```python
from build123d import *

# Parameters (mm, degrees)
BOSS_EXTRU_1_DEPTH      = 5
ENL_V_MAT_EXTRU_1_REACH = 7


with BuildPart() as part:
    # Esquisse1 → Boss.-Extru.1 (new body)
    with BuildSketch(Plane.XY):
        Polygon((0, 0), (0, 15), (-5, 15), (-5, 55), (0, 55), (0, 80), (490, 80), (490, 55), (495, 55), (495, 15), (490, 15), (490, 0), align=None)
    extrude(amount=BOSS_EXTRU_1_DEPTH)

    # Esquisse2 → Enlèv. mat.-Extru.1 (cut, up to next)
    with BuildSketch(Plane.XY.offset(5), mode=Mode.PRIVATE) as enl_v_mat_extru_1_sk1:
        with BuildLine():
            Line((35, 25), (455, 25))
            ThreePointArc((455, 25), (462.071067812, 27.928932188), (465, 35))
            Line((465, 35), (465, 45))
            ThreePointArc((465, 45), (462.071067812, 52.071067812), (455, 55))
            Line((455, 55), (35, 55))
            ThreePointArc((35, 55), (27.928932188, 52.071067812), (25, 45))
            Line((25, 45), (25, 35))
            ThreePointArc((25, 35), (27.928932188, 27.928932188), (35, 25))
        make_face()
    enl_v_mat_extru_1_tool1 = extrude(enl_v_mat_extru_1_sk1.sketch, amount=-ENL_V_MAT_EXTRU_1_REACH, mode=Mode.PRIVATE) & part.part
    add(enl_v_mat_extru_1_tool1.solids().sort_by_distance((245, 40, 5))[0], mode=Mode.SUBTRACT)


solid = part.part
```
Verification items for the finished model (mm, model axes). A direction names the side the tool comes from. Round coordinates to 2 decimals unless told otherwise and drop trailing zeros. Loops run counter-clockwise (first coordinate to the right, second up) from the corner with the lowest first, then second, coordinate; pieces in that order, holes last. Notation, with made-up numbers: (84.25, 69) -> (136.25, 69) arc R34 ccw to (136.25, 103) -> close; hole circle Ø9 at (-18, 74). An arc over 180 degrees is marked (long way). Answer as a JSON object with one key per item and string values.
Q1. Draft check along Y on faces 3 (the cylindrical face through (462.15, 51.99, 2.54)), 4 (the flat face through (248, 58, 0)). Enter one of: pulls with the +Y half, pulls with the -Y half, needs draft (parallel to the pull), parting line crosses it, or undercut.
Data:
{"face 3": "undercut", "face 4": "needs draft"}
Q2. Scan lines: line 1 (X direction, y = 41, z = 2.5); line 2 (Y direction, x = 366.5, z = 4.1); line 3 (X direction, y = 65.5, z = 3.8). Record each from-to range of solid material in increasing order. Write a range as from..to.
Data:
{"line 1": "x = -5..25, 465..495", "line 2": "y = 0..25, 55..80", "line 3": "x = 0..490"}
Q3. Section check B-B (z = 3.75). Record the boundary of the cut face in (x, y).
Data:
{"outline": "(-5, 15) -> (0, 15) -> (0, 0) -> (490, 0) -> (490, 15) -> (495, 15) -> (495, 55) -> (490, 55) -> (490, 80) -> (0, 80) -> (0, 55) -> (-5, 55) -> close; hole (25, 35) arc R10 ccw to (35, 25) -> (455, 25) arc R10 ccw to (465, 35) -> (465, 45) arc R10 ccw to (455, 55) -> (35, 55) arc R10 ccw to (25, 45) -> close"}
Q4. Go/stop test with flat-tipped pins: P1, Ø1.5, axis at y = 71, z = 2, coming from the -X side; P2, Ø1.5, axis at y = 4, z = 3.5, coming from the +X side. Record where each tip stops, or that it passes through.
Data:
{"P1": "stops at x = 0", "P2": "stops at x = 490"}
Q5. Section check A-A (x = 325). Record the boundary of the cut face in (y, z).
Data:
{"outline": "(0, 0) -> (25, 0) -> (25, 5) -> (0, 5) -> close; (55, 0) -> (80, 0) -> (80, 5) -> (55, 5) -> close"}
Q6. Section check C-C (y = 70.5). Record the boundary of the cut face in (x, z), then the cut area to 3 significant figures.
Data:
{"outline": "(0, 0) -> (490, 0) -> (490, 5) -> (0, 5) -> close", "area": "2,450 mm2"}
Q7. Access from +Z, -Z, +X, -X, +Y, -Y to the whole of each face (thin tool, end or side, straight path). Record for faces 1 (the flat face through (248, 58, 5)), 2 (the cylindrical face through (27.85, 28.01, 2.54)).
Data:
{"face 1": "+Z, +X, -X, +Y, -Y", "face 2": "+Z, -Z"}
